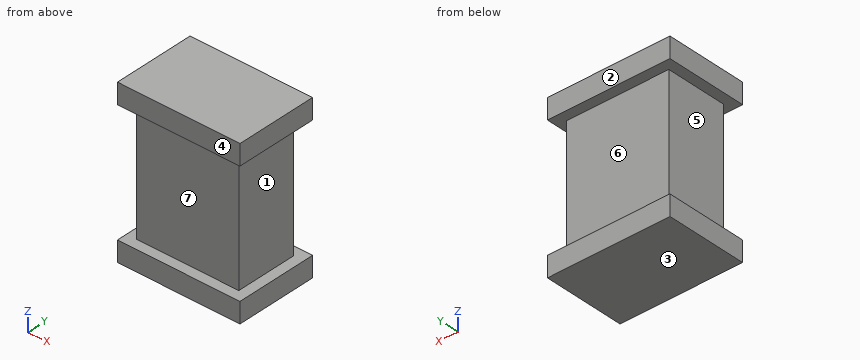
from build123d import *

# Parameters (mm, degrees)
F0_W     = 5
F0_H     = 3
F1_DEPTH = 6
F2_W     = 6
F2_H     = 4
F3_DEPTH = 1
F4_W     = 6
F4_H     = 4
F5_DEPTH = 1


with BuildPart() as f1:
    # F0 (on Top) → F1 (new body)
    with BuildSketch(Plane.XY):
        Rectangle(F0_W, F0_H)
    extrude(amount=F1_DEPTH)

    # F2 (on face) → F3 (join)
    with BuildSketch(Plane.XY.offset(6)):
        Rectangle(F2_W, F2_H)
    extrude(amount=F3_DEPTH)

    # F4 (on face) → F5 (join)
    with BuildSketch(Plane(origin=(0, 0, 0), x_dir=(1, 0, 0), z_dir=(0, 0, -1))):
        Rectangle(F4_W, F4_H)
    extrude(amount=F5_DEPTH)


solid = f1.part
Input: part model. Units: mm. Frame: model coordinates. Face numbers are marked on the shaded views. A direction names the side the tool comes from. Coordinates: 2 decimals unless noted, no trailing zeros. Loops run counter-clockwise (first coordinate to the right, second up) from the corner with the lowest first, then second, coordinate; pieces in that order, holes last.
(1) Material intervals for probe 1 along Z at (x, y) = (2.7, -0.5); probe 2 along X at (y, z) = (-1, 3.75); probe 3 along Y at (x, z) = (-1.2, 5), sorted ascending.
(2) Section D-D on z = 2.75. Return the cut outline in (x, y).
(3) First-contact query: pin 1 Ø2 at (x, z) = (-2, 3) entering from +Y. Flat tip, straight axial feed; report the tip coordinate or a pass-through.
(4) Section A-A on y = -1.7. Return the cut outline in (x, z), then the cut area to 3 significant figures.
(5) Pull-direction query (Z, two-part tool) for the marked faces 1, 2 and 3; classes: released by +Z, released by -Z, zero draft, split by the parting line, or undercut.
(6) Set-up query: the marked faces 4, 5, 6 and 7. Return all of +Z, -Z, +X, -X, +Y, -Y with unobstructed straight access to the full face (end or side cutting, diameter ignored); none if empty.
(7) Section B-B on x = 1.1. Return the cut outline in (y, z).
(8) Section C-C on y = -0.5. Return the cut outline in (x, z), then the cut area to 3 significant figures.
Data:
1. probe 1: z = -1 to 0, 6 to 7
1. probe 2: x = -2.5 to 2.5
1. probe 3: y = -1.5 to 1.5
2. outline: (-2.5, -1.5) - (2.5, -1.5) - (2.5, 1.5) - (-2.5, 1.5) - close
3. pin 1: stops at y = 1.5
4. outline: (-3, -1) - (3, -1) - (3, 0) - (-3, 0) - close; (-3, 6) - (3, 6) - (3, 7) - (-3, 7) - close
4. area: 12.0 mm2
5. face 1: undercut
5. face 2: zero draft
5. face 3: released by -Z
6. face 4: +Z, -Z, +X, -X, -Y
6. face 5: -X, +Y, -Y
6. face 6: +X, -X, +Y
6. face 7: +X, -X, -Y
7. outline: (-2, -1) - (2, -1) - (2, 0) - (1.5, 0) - (1.5, 6) - (2, 6) - (2, 7) - (-2, 7) - (-2, 6) - (-1.5, 6) - (-1.5, 0) - (-2, 0) - close
8. outline: (-3, -1) - (3, -1) - (3, 0) - (2.5, 0) - (2.5, 6) - (3, 6) - (3, 7) - (-3, 7) - (-3, 6) - (-2.5, 6) - (-2.5, 0) - (-3, 0) - close
8. area: 42.0 mm2
